Check sheet for the drawn part. Datum: minimum x, y, z corner. Units: mm. Coordinates: 2 decimals unless noted, no trailing zeros. Write each loop counter-clockwise with the first axis right and the second up, starting at its lowest first coordinate (ties: lowest second). Pieces come first, ordered by that corner, then holes. Notation, with made-up numbers: M -19,60.5 L 6,60.5 A32 cw 6,99.5 Z; hole C -11.5,-23 d5. An arc over 180 degrees is marked long. Answer in a Markdown table with one row per item.
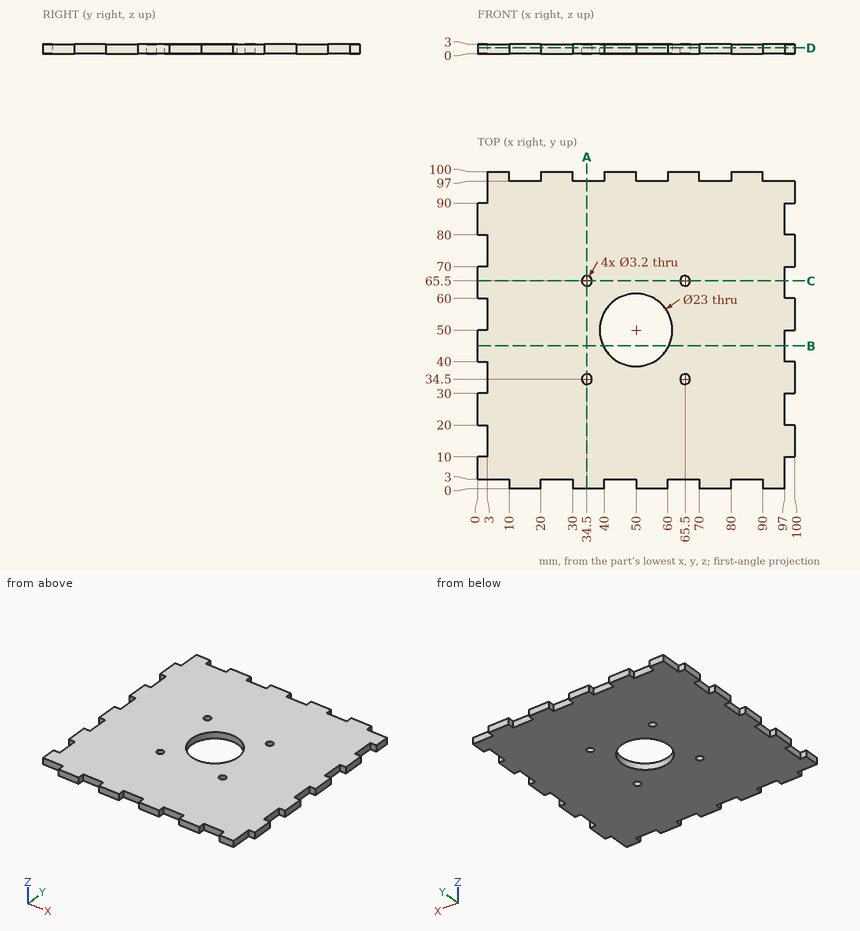
1) Sectioned sample at B-B (y = 45). Record the cut outline in (x, z), then the cut area to 3 significant figures.
Response values:
| item | result |
|---|---|
| outline | M 0,0 L 39.64,0 L 39.64,3 L 0,3 Z; M 60.36,0 L 97,0 L 97,3 L 60.36,3 Z |
| area | 229 mm² |
2) Sectioned sample at A-A (x = 34.5). Record the cut outline in (y, z), then the cut area to 3 significant figures.
Response values:
| item | result |
|---|---|
| outline | M 0,0 L 32.9,0 L 32.9,3 L 0,3 Z; M 36.1,0 L 63.9,0 L 63.9,3 L 36.1,3 Z; M 67.1,0 L 97,0 L 97,3 L 67.1,3 Z |
| area | 272 mm² |
3) Depth check by flat-ended pin: pin 1 (0.9 mm diameter, centred on y = 98, z = 2, fed in from +X); pin 2 (3 mm diameter, centred on x = 65.5, y = 34.5, fed in from -Z); pin 3 (0.9 mm diameter, centred on y = 17, z = 2, fed in from -X); pin 4 (0.9 mm diameter, centred on x = 99, z = 1.5, fed in from +Y). Enter the tip coordinate at first touch or a pass-through.
Response values:
| item | result |
|---|---|
| pin 1 | stops at x = 90 |
| pin 2 | passes through |
| pin 3 | stops at x = 3 |
| pin 4 | stops at y = 97 |
4) Thickness scan on L1, parallel to Y at x = 34.5, z = 1.65; L2, parallel to Y at x = 65.5, z = 1.5; L3, parallel to X at y = 66.5, z = 0.6. Record the ranges inside material, lowest first. Write a range as [from, to].
Response values:
| item | result |
|---|---|
| L1 | y = [0, 32.9], [36.1, 63.9], [67.1, 97] |
| L2 | y = [3, 32.9], [36.1, 63.9], [67.1, 100] |
| L3 | x = [0, 33.25], [35.75, 64.25], [66.75, 97] |
5) Sectioned sample at D-D (z = 1.8). Give the number of separate pieces and of enclosed holes in the cut face, then the cut area to 3 significant figures.
Response values:
| item | result |
|---|---|
| separate pieces | 1 |
| enclosed holes | 5 |
| area | 8,950 mm² |
